Autodesk Inventor part; units mm, degrees
ref_plane "YZ Plane" through (0, 0, 0) normal (1, 0, 0) x (0, 1, 0)
ref_plane "XZ Plane" through (0, 0, 0) normal (0, 1, 0) x (-1, 0, 0)
ref_plane "XY Plane" through (0, 0, 0) normal (0, 0, 1) x (1, 0, 0)
sketch "Sketch1" plane through (0, 0, 0) normal (0, 0, 1) x (1, 0, 0)
  line L0 (36, -20) -> (-36, -20) construction
  line L1 (-36, -20) -> (-36, 20) construction
  line L2 (-36, 20) -> (36, 20) construction
  line L3 (36, 20) -> (36, -20) construction
  line L4 (36, -20) -> (-36, 20) construction
  line L5 (-36, -20) -> (36, 20) construction
  line L6 (42.35, -26.35) -> (-42.35, -26.35)
  line L7 (-42.35, -26.35) -> (-42.35, 26.35)
  line L8 (-42.35, 26.35) -> (42.35, 26.35)
  line L9 (42.35, 26.35) -> (42.35, -26.35)
  line L10 (42.35, -26.35) -> (-42.35, 26.35) construction
  line L11 (-42.35, -26.35) -> (42.35, 26.35) construction
  point P0 (0, 0)
  dimension "d0" = 72
  dimension "d1" = 40
  dimension "d2" = 6.35
  dimension "d3" = 6.35
extrude "Extrusion1" add sketch "Sketch1" along normal blind 6.35
sketch "Sketch2" plane through (42.35, -26.35, 0) normal (1, 0, 0) x (0, 0, -1)
  line L0 (-6.35, 0) -> (-6.35, 52.7)
  line L1 (-6.35, 52.7) -> (-50.5706, 0)
  line L2 (-50.5706, 0) -> (-6.35, 0)
  point P0 (0, 26.35)
  dimension "d13" = 40
extrude "Extrusion2" add sketch "Sketch2" against normal up to surface (84.7 mm away)
hole "Hole2" at (-36, 20, 0) at (-36, -20, 0) at (36, -20, 0) at (36, 20, 0) direction (0, 0, 1) diameter 5.1054 end through all
properties part number "limelight mount" material "ABS Plastic"
Could you check a few things on this model? Use its own coordinates, in mm. Give positions to 0.01 mm unless a question says otherwise; leave off trailing zeros. Order: outer loops, then holes, each group sorted by start corner. A loop starts at its lowest first (then second) coordinate and runs counter-clockwise, first axis right, second up. Notation, with made-up numbers: (3.5, 40.5) - (58.5, 40.5) arc R9 ccw to (58.5, 51.5) - close; hole circle Ø3 at (27.5, -20). An arc over 180 degrees is marked (long way). One line per question, with ' | ' between items. Start each with the question number.
Item 1: Thinking about a two-plate mould opening in Y: for faces 1 (the flat face through (1, -26.35, 25)), 2 (the flat face through (-1, 0, 0)), 3 (the cylindrical face through (-36.11, -22.55, 24.04)), 4 (the cylindrical face through (-36.11, 17.45, 5.48)), which applies, pulls with the +Y half, pulls with the -Y half, needs draft (parallel to the pull), parting line crosses it, or undercut?
Item 2: I want a section at B-B on y = -20. Write out the boundary of the cut face in (x, z).
Item 3: I'm going to push flat-ended pins straight in: pin 1 Ø8 at (x, y) = (-36, 20) entering from +Z; pin 2 Ø3 at (x, y) = (36, -20) entering from -Z; pin 3 Ø12 at (x, y) = (-21, 9.5) entering from +Z; pin 4 Ø8 at (x, z) = (-0.5, 22.5) entering from +Y. Where does each tip first touch, or does it pass through?
Item 4: I want a section at A-A on z = 4.5. Write out the boundary of the cut face in (x, y).
Item 5: I need wall thicknesses on probe 1 along X at (y, z) = (-20, 16.5); probe 2 along Y at (x, z) = (-36, 3.25); probe 3 along X at (y, z) = (-19.5, 11). Which ranges of each line are inside material? Lowest first, please. Write a range as [from, to].
Item 6: I want a section at C-C on z = 12. Write out the boundary of the cut face in (x, y).
Item 7: I want a section at D-D on x = 36. Write out the boundary of the cut face in (y, z).
Verdict:
1) face 1: pulls with the -Y half | face 2: needs draft | face 3: undercut | face 4: undercut
2) outline: (-42.35, 0) - (-38.55, 0) - (-38.55, 45.24) - (-42.35, 45.24) - close; (-33.45, 0) - (33.45, 0) - (33.45, 45.24) - (-33.45, 45.24) - close; (38.55, 0) - (42.35, 0) - (42.35, 45.24) - (38.55, 45.24) - close
3) pin 1: z = 15.03 | pin 2: through | pin 3: z = 25.52 | pin 4: y = 11.87
4) outline: (-42.35, -26.35) - (42.35, -26.35) - (42.35, 26.35) - (-42.35, 26.35) - close; hole circle Ø5.11 at (-36, -20); hole circle Ø5.11 at (-36, 20); hole circle Ø5.11 at (36, -20); hole circle Ø5.11 at (36, 20)
5) probe 1: [-42.35, -38.55], [-33.45, 33.45], [38.55, 42.35] | probe 2: [-26.35, -22.55], [-17.45, 17.45], [22.55, 26.35] | probe 3: [-42.35, -38.5], [-33.5, 33.5], [38.5, 42.35]
6) outline: (-42.35, -26.35) - (42.35, -26.35) - (42.35, 19.62) - (38.52, 19.62) arc R2.55 cw to (33.48, 19.62) - (-33.48, 19.62) arc R2.55 cw to (-38.52, 19.62) - (-42.35, 19.62) - close; hole circle Ø5.11 at (-36, -20); hole circle Ø5.11 at (36, -20)
7) outline: (-26.35, 0) - (-22.55, 0) - (-22.55, 47.38) - (-26.35, 50.57) - close; (-17.45, 0) - (17.45, 0) - (17.45, 13.82) - (-17.45, 43.1) - close; (22.55, 0) - (26.35, 0) - (26.35, 6.35) - (22.55, 9.54) - close
